Could you check a few things on this drawing? It's one solid part, dimensions in mm from its lowest x, y, z. Give positions to 0.01 mm unless a question says otherwise; leave off trailing zeros. Order: outer loops, then holes, each group sorted by start corner. A loop starts at its lowest first (then second) coordinate and runs counter-clockwise, first axis right, second up. Notation, with made-up numbers: (38.25, 37) -> (60.25, 37) arc R19 cw to (60.25, 66) -> close; hole circle Ø7 at (50, 70). An arc over 180 degrees is marked (long way). Write each question's results on one line, items separated by ' | '. Start each with the question number.
Q1. Imagine slicing it at C-C, the plane z = 35.5. Please give me the cut outline in (x, y), then the cut area to 3 significant figures.
Q2. Imagine slicing it at D-D, the plane x = 79.5. Please give me the cut outline in (y, z) (1 decimal).
Q3. Thinking about a two-plate mould opening in X: for the marked faces 1, 2 and 3, which applies, pulls with the +X half, pulls with the -X half, needs draft (parallel to the pull), parting line crosses it, or undercut?
Q4. I'm going to push flat-ended pins straight in: pin 1 (5 mm diameter, centred on x = 201.5, y = 145.5, fed in from +Z); pin 2 (1.5 mm diameter, centred on x = 192.5, z = 84, fed in from -Y) (1 decimal); pin 3 (10 mm diameter, centred on x = 136.5, z = 42, fed in from -Y). Where does each tip first touch, or does it pass through?
Q5. Imagine slicing it at A-A, the plane y = 160. Please give me the cut outline in (x, z), then the cut area to 3 significant figures.
Q6. I need wall thicknesses on line 1 along Y through (x, z) = (160, 8); line 2 along Z through (x, y) = (282, 138.5); line 3 along X through (y, z) = (159, 85.5) (1 decimal). Which ranges of each line are inside material? Lowest first, please. Write a range as [from, to].
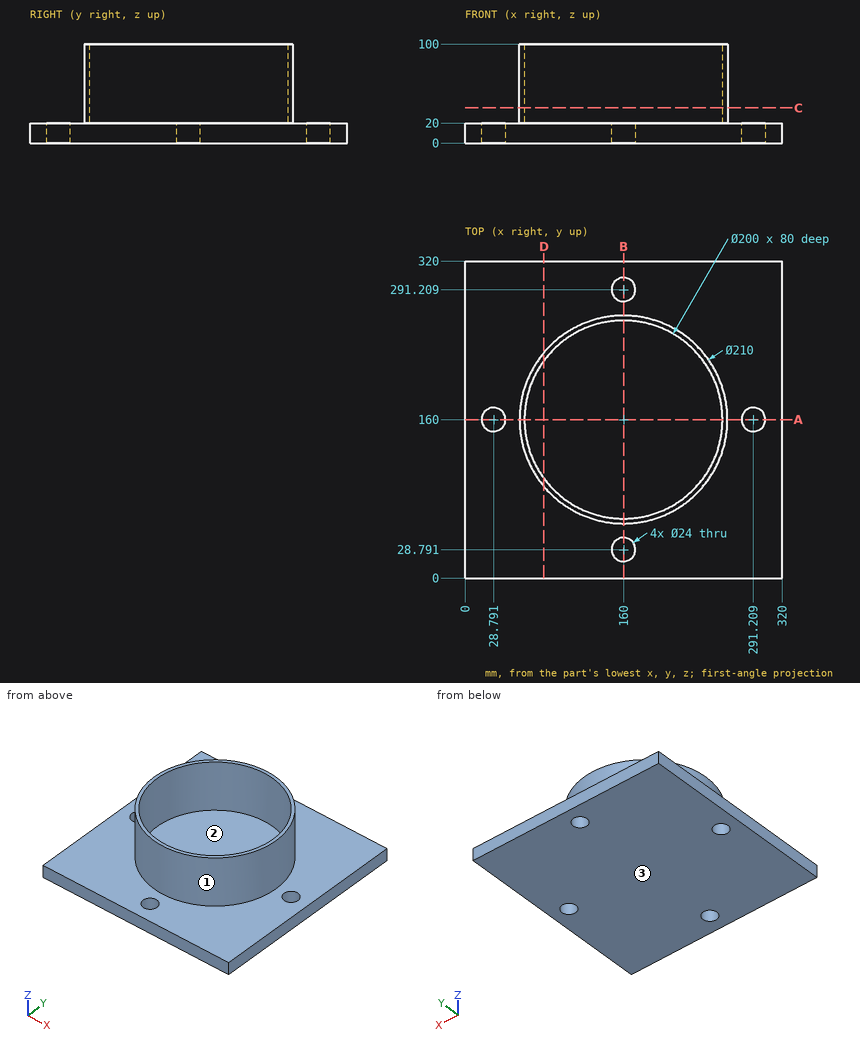
Geometry check:
1) outline: circle Ø210 at (160, 160); hole circle Ø200 at (160, 160) | area: 3,220 mm²
2) outline: (0, 0) -> (320, 0) -> (320, 20) -> (227.4, 20) -> (227.4, 100) -> (219.3, 100) -> (219.3, 20) -> (100.7, 20) -> (100.7, 100) -> (92.6, 100) -> (92.6, 20) -> (0, 20) -> close
3) face 1: parting line crosses it | face 2: undercut | face 3: needs draft
4) pin 1: z = 20 | pin 2: y = 59.9 | pin 3: y = 56.64
5) outline: (0, 0) -> (16.79, 0) -> (16.79, 20) -> (0, 20) -> close; (40.79, 0) -> (279.21, 0) -> (279.21, 20) -> (265, 20) -> (265, 100) -> (260, 100) -> (260, 20) -> (60, 20) -> (60, 100) -> (55, 100) -> (55, 20) -> (40.79, 20) -> close; (303.21, 0) -> (320, 0) -> (320, 20) -> (303.21, 20) -> close | area: 6,240 mm²
6) line 1: [0, 16.79], [40.79, 279.21], [303.21, 320] | line 2: [0, 20] | line 3: [55, 60], [260, 265]
